```python
from build123d import *

# Parameters (mm, degrees)
SKETCH1_W           = 150
SKETCH1_H           = 53.34
BOSS_EXTRUDE1_DEPTH = 10
SKETCH4_W           = 150
SKETCH4_H           = 10.16
BOSS_EXTRUDE3_DEPTH = 127
CUT_EXTRUDE1_DEPTH  = 83.82
FILLET1_R           = 2.54
SKETCH7_R           = 4.649830258
CUT_EXTRUDE2_DEPTH  = 83.82
SKETCH8_W           = 53.10558352
SKETCH8_H           = 45.72
CUT_EXTRUDE3_DEPTH  = 12.7
CUT_EXTRUDE4_DEPTH  = 157.841179542
FILLET2_R           = 2.54
FILLET3_R           = 2.54
CUT_EXTRUDE5_REACH  = 160.446
SKETCH10_R          = 1.7
SKETCH11_R          = 4.699
CUT_EXTRUDE6_DEPTH  = 157.841179542


with BuildPart() as part:
    # Sketch1 → Boss-Extrude1 (new body)
    with BuildSketch(Plane.XY):
        Rectangle(SKETCH1_W, SKETCH1_H)
    extrude(amount=BOSS_EXTRUDE1_DEPTH)

    # Sketch4 → Boss-Extrude3 (add)
    with BuildSketch(Plane(origin=(0, 0, 0), x_dir=(-1, 0, 0), z_dir=(0, 0, -1))):
        with Locations((0, 21.59)):
            Rectangle(SKETCH4_W, SKETCH4_H)
        with Locations((0, -21.59)):
            Rectangle(SKETCH4_W, SKETCH4_H)
    extrude(amount=BOSS_EXTRUDE3_DEPTH)

    # Sketch6 → Cut-Extrude1 (cut)
    with BuildSketch(Plane(origin=(0, 26.67, 0), x_dir=(1, 0, 0), z_dir=(0, 1, 0))):
        Polygon((28.775780248, 127), (75, 0), (75, 127), align=None)
        Polygon((-75, 0), (-75, 127), (-28.775780248, 127), align=None)
    extrude(amount=-CUT_EXTRUDE1_DEPTH, mode=Mode.SUBTRACT)

    # Fillet1
    fillet1_edges = [part.edges().sort_by_distance(p)[0] for p in [
        (28.775780248, 21.59, -127),
        (-28.775780248, 21.59, -127),
        (-28.775780248, -21.59, -127),
        (28.775780248, -21.59, -127),
    ]]
    fillet(fillet1_edges, radius=FILLET1_R)

    # Sketch7 → Cut-Extrude2 (cut)
    with BuildSketch(Plane(origin=(0, 26.67, 0), x_dir=(1, 0, 0), z_dir=(0, 1, 0))):
        with Locations(Location((0, 114.3, 0), (0, 0, 270))):
            Circle(SKETCH7_R)
    extrude(amount=-CUT_EXTRUDE2_DEPTH, mode=Mode.SUBTRACT)

    # Sketch8 → Cut-Extrude3 (cut)
    with BuildSketch(Plane.XY.offset(10)):
        Rectangle(SKETCH8_W, SKETCH8_H)
    extrude(amount=-CUT_EXTRUDE3_DEPTH, mode=Mode.SUBTRACT)

    # Sketch9 → Cut-Extrude4 (cut, through all)
    with BuildSketch(Plane(origin=(0, 26.67, 0), x_dir=(1, 0, 0), z_dir=(0, 1, 0))):
        Polygon((-34.586424408, 93.969139079), (-9.684580109, 111.082069913), (-25.640652678, 120.607649188), align=None)
        Polygon((-39.704336807, 78.729139079), (-10.827990436, 95.842069913), (-10.827990436, 67.313152305), align=None)
        Polygon((-10.827990436, 52.073152305), (-44.822249205, 63.489139079), (-56.460793416, 28.832153973), align=None)
        Polygon((-10.827990436, 36.833152305), (-61.578705814, 13.592153973), (-10.827990436, 13.592153973), align=None)
    cut_extrude4 = extrude(amount=-CUT_EXTRUDE4_DEPTH, mode=Mode.SUBTRACT)

    # Mirror1: Cut-Extrude4 across plane
    add(cut_extrude4.mirror(Plane(origin=(0, 0, 0), x_dir=(0, 0, 1), z_dir=(1, 0, 0))), mode=Mode.SUBTRACT)

    # Fillet2
    fillet2_edges = [part.edges().sort_by_distance(p)[0] for p in [
        (-10.827990436, 21.59, -67.313152305),
        (-39.704336807, -21.59, -78.729139079),
        (-39.704336807, 21.59, -78.729139079),
        (-10.827990436, 21.59, -95.842069913),
        (-10.827990436, 21.59, -52.073152305),
        (-56.460793416, 21.59, -28.832153973),
        (-44.822249205, 21.59, -63.489139079),
        (-10.827990436, 21.59, -36.833152305),
        (-10.827990436, 21.59, -13.592153973),
        (-61.578705814, 21.59, -13.592153973),
        (-34.586424408, 21.59, -93.969139079),
        (-25.640652678, 21.59, -120.607649188),
        (-9.684580109, 21.59, -111.082069913),
        (39.704336807, 21.59, -78.729139079),
        (10.827990436, 21.59, -67.313152305),
        (10.827990436, 21.59, -95.842069913),
        (56.460793416, 21.59, -28.832153973),
        (10.827990436, 21.59, -52.073152305),
        (44.822249205, 21.59, -63.489139079),
        (10.827990436, 21.59, -13.592153973),
        (10.827990436, 21.59, -36.833152305),
        (61.578705814, 21.59, -13.592153973),
        (25.640652678, 21.59, -120.607649188),
        (34.586424408, 21.59, -93.969139079),
        (9.684580109, -21.59, -111.082069913),
        (9.684580109, 21.59, -111.082069913),
    ]]
    fillet(fillet2_edges, radius=FILLET2_R)

    # Fillet3
    fillet3_edges = [part.edges().sort_by_distance(p)[0] for p in [
        (-10.827990436, -21.59, -67.313152305),
        (-10.827990436, -21.59, -95.842069913),
        (-10.827990436, -21.59, -52.073152305),
        (-56.460793416, -21.59, -28.832153973),
        (-44.822249205, -21.59, -63.489139079),
        (-10.827990436, -21.59, -36.833152305),
        (-10.827990436, -21.59, -13.592153973),
        (-61.578705814, -21.59, -13.592153973),
        (-34.586424408, -21.59, -93.969139079),
        (-25.640652678, -21.59, -120.607649188),
        (-9.684580109, -21.59, -111.082069913),
        (39.704336807, -21.59, -78.729139079),
        (10.827990436, -21.59, -67.313152305),
        (10.827990436, -21.59, -95.842069913),
        (56.460793416, -21.59, -28.832153973),
        (10.827990436, -21.59, -52.073152305),
        (44.822249205, -21.59, -63.489139079),
        (10.827990436, -21.59, -13.592153973),
        (10.827990436, -21.59, -36.833152305),
        (61.578705814, -21.59, -13.592153973),
        (25.640652678, -21.59, -120.607649188),
        (34.586424408, -21.59, -93.969139079),
    ]]
    fillet(fillet3_edges, radius=FILLET3_R)

    # Sketch10 → Cut-Extrude5 (cut, up to next)
    with BuildSketch(Plane.XY.offset(10), mode=Mode.PRIVATE) as cut_extrude5_sk1:
        with Locations((40.113762047, 9.239336029)):
            Circle(SKETCH10_R)
    cut_extrude5_tool1 = extrude(cut_extrude5_sk1.sketch, amount=-CUT_EXTRUDE5_REACH, mode=Mode.PRIVATE) & part.part
    # Sketch10 → Cut-Extrude5 (cut, up to next)
    with BuildSketch(Plane.XY.offset(10), mode=Mode.PRIVATE) as cut_extrude5_sk2:
        with Locations((64.827817703, 9.239336029)):
            Circle(SKETCH10_R)
    cut_extrude5_tool2 = extrude(cut_extrude5_sk2.sketch, amount=-CUT_EXTRUDE5_REACH, mode=Mode.PRIVATE) & part.part
    # Sketch10 → Cut-Extrude5 (cut, up to next)
    with BuildSketch(Plane.XY.offset(10), mode=Mode.PRIVATE) as cut_extrude5_sk3:
        with Locations((64.827817703, -13.049336029)):
            Circle(SKETCH10_R)
    cut_extrude5_tool3 = extrude(cut_extrude5_sk3.sketch, amount=-CUT_EXTRUDE5_REACH, mode=Mode.PRIVATE) & part.part
    # Sketch10 → Cut-Extrude5 (cut, up to next)
    with BuildSketch(Plane.XY.offset(10), mode=Mode.PRIVATE) as cut_extrude5_sk4:
        with Locations((40.113762047, -13.049336029)):
            Circle(SKETCH10_R)
    cut_extrude5_tool4 = extrude(cut_extrude5_sk4.sketch, amount=-CUT_EXTRUDE5_REACH, mode=Mode.PRIVATE) & part.part
    # Sketch10 → Cut-Extrude5 (cut, up to next)
    with BuildSketch(Plane.XY.offset(10), mode=Mode.PRIVATE) as cut_extrude5_sk5:
        with Locations((-60.450241723, 9.239336029)):
            Circle(SKETCH10_R)
    cut_extrude5_tool5 = extrude(cut_extrude5_sk5.sketch, amount=-CUT_EXTRUDE5_REACH, mode=Mode.PRIVATE) & part.part
    # Sketch10 → Cut-Extrude5 (cut, up to next)
    with BuildSketch(Plane.XY.offset(10), mode=Mode.PRIVATE) as cut_extrude5_sk6:
        with Locations((-35.736186067, 9.239336029)):
            Circle(SKETCH10_R)
    cut_extrude5_tool6 = extrude(cut_extrude5_sk6.sketch, amount=-CUT_EXTRUDE5_REACH, mode=Mode.PRIVATE) & part.part
    # Sketch10 → Cut-Extrude5 (cut, up to next)
    with BuildSketch(Plane.XY.offset(10), mode=Mode.PRIVATE) as cut_extrude5_sk7:
        with Locations((-35.736186067, -13.049336029)):
            Circle(SKETCH10_R)
    cut_extrude5_tool7 = extrude(cut_extrude5_sk7.sketch, amount=-CUT_EXTRUDE5_REACH, mode=Mode.PRIVATE) & part.part
    # Sketch10 → Cut-Extrude5 (cut, up to next)
    with BuildSketch(Plane.XY.offset(10), mode=Mode.PRIVATE) as cut_extrude5_sk8:
        with Locations((-60.450241723, -13.049336029)):
            Circle(SKETCH10_R)
    cut_extrude5_tool8 = extrude(cut_extrude5_sk8.sketch, amount=-CUT_EXTRUDE5_REACH, mode=Mode.PRIVATE) & part.part
    add(cut_extrude5_tool1.solids().sort_by_distance((40.113762, 9.239336, 10))[0], mode=Mode.SUBTRACT)
    add(cut_extrude5_tool2.solids().sort_by_distance((64.827818, 9.239336, 10))[0], mode=Mode.SUBTRACT)
    add(cut_extrude5_tool3.solids().sort_by_distance((64.827818, -13.049336, 10))[0], mode=Mode.SUBTRACT)
    add(cut_extrude5_tool4.solids().sort_by_distance((40.113762, -13.049336, 10))[0], mode=Mode.SUBTRACT)
    add(cut_extrude5_tool5.solids().sort_by_distance((-60.450242, 9.239336, 10))[0], mode=Mode.SUBTRACT)
    add(cut_extrude5_tool6.solids().sort_by_distance((-35.736186, 9.239336, 10))[0], mode=Mode.SUBTRACT)
    add(cut_extrude5_tool7.solids().sort_by_distance((-35.736186, -13.049336, 10))[0], mode=Mode.SUBTRACT)
    add(cut_extrude5_tool8.solids().sort_by_distance((-60.450242, -13.049336, 10))[0], mode=Mode.SUBTRACT)

    # Sketch11 → Cut-Extrude6 (cut, through all)
    with BuildSketch(Plane(origin=(0, 26.67, 0), x_dir=(1, 0, 0), z_dir=(0, 1, 0))):
        with Locations(Location((0, 50.739787161, 0), (0, 0, 270))):
            Circle(SKETCH11_R)
    extrude(amount=-CUT_EXTRUDE6_DEPTH, mode=Mode.SUBTRACT)


solid = part.part
```
Work out the finished part from the listing and answer in its coordinate system (mm). A direction names the side the tool comes from. Give positions to 0.01 mm unless a question says otherwise; leave off trailing zeros. Loops run counter-clockwise (first coordinate to the right, second up) from the corner with the lowest first, then second, coordinate; pieces in that order, holes last. Notation, with made-up numbers: (69, 4) -> (103, 4) arc R25 ccw to (103, 18) -> close; hole circle Ø6 at (30.25, 89.5). An arc over 180 degrees is marked (long way). One line per question, with ' | ' between items. Start each with the question number.
1) Section B-B, the plane x = 7 is taken. Determine the outline of the cut face in (y, z), then the cut area to 3 significant figures.
2) Each of these flat-tipped pins is pushed along its axis until it touches: pin 1 (3 mm diameter, centred on y = 21.5, z = -25, fed in from +X); pin 2 (5 mm diameter, centred on y = -21.5, z = -84, fed in from -X); pin 3 (4.5 mm diameter, centred on x = -35.74, y = 9.24, fed in from -Z); pin 4 (4 mm diameter, centred on x = -60.45, y = 9.24, fed in from +Z). Where does it stop, or does it pass through?
3) Determine the mould class of faces 4 (the face through (38.765, 8.205, 5.07)), 5 (the face through (-24.45, 21.66, -72.7)) for opening direction Y: +Y half, -Y half, draft (parallel to the pull), parting line (faces both ways), or undercut.
4) For faces 1 (the face through (0, -22.86, 4)), 2 (the face through (38.76, -14.08, 5.07)), 3 (the face through (25.1, 21.5, -119.2)), determine the directions among +Z, -Z, +X, -X, +Y, -Y from which every point of the face is accessible in a straight line to the end or side of a thin tool.
5) Straight lines are drawn through the part: L1, parallel to Y at x = 9, z = -110; L2, parallel to X at y = -21, z = -114; L3, parallel to X at y = 4.5, z = 1.5. For each, find the intervals that lie inside material, in ascending order.
6) Section C-C, the plane x = 61 is taken. Determine the outline of the cut face in (y, z), then the cut area to 4 significant figures.
7) Section A-A, the plane y = -6.5 is taken. Determine the outline of the cut face in (x, z), then the cut area to 3 significant figures.
Resolved:
1) outline: (-26.67, -127) -> (-16.51, -127) -> (-16.51, -2.7) -> (-22.86, -2.7) -> (-22.86, 10) -> (-26.67, 10) -> close; (16.51, -127) -> (26.67, -127) -> (26.67, 10) -> (22.86, 10) -> (22.86, -2.7) -> (16.51, -2.7) -> close | area: 2,620 mm2
2) pin 1: x = 66.45 | pin 2: x = -45.34 | pin 3: z = 0 | pin 4: z = 10
3) face 4: undercut | face 5: draft
4) face 1: +Z | face 2: +Z, -Z | face 3: +Y, -Y
5) L1: -26.67 to -16.51, 16.51 to 26.67 | L2: -33.51 to -27.86, -14.57 to -4.64, 4.64 to 14.57, 27.86 to 33.51 | L3: -75 to -26.55, 26.55 to 75
6) outline: (-26.67, -38.46) -> (-16.51, -38.46) -> (-16.51, 0) -> (16.51, 0) -> (16.51, -38.46) -> (26.67, -38.46) -> (26.67, 10) -> (-26.67, 10) -> close | area: 1,315 mm2
7) outline: (-75, 0) -> (-26.55, 0) -> (-26.55, 10) -> (-75, 10) -> close; (26.55, 0) -> (75, 0) -> (75, 10) -> (26.55, 10) -> close | area: 969 mm2
